Check sheet for the modelled part. Datum: model origin and axes. Units: mm. A direction names the side the tool comes from. Coordinates: 2 decimals unless noted, no trailing zeros. Loops run counter-clockwise (first coordinate to the right, second up) from the corner with the lowest first, then second, coordinate; pieces in that order, holes last.
```python
from build123d import *

# Parameters (mm, degrees)
F0_R     = 6
F1_DEPTH = 16
F2_R     = 2
F3_DEPTH = 12.5
F4_R     = 4
F5_DEPTH = 12


# Not quite as in the source:
# - a fillet or chamfer that OpenCascade refuses, or shapes differently, is made with other operations: its cross-section is extruded or revolved along the edge and cut away or added


with BuildPart() as f1:
    # F0 (on Top) → F1 (new body)
    with BuildSketch(Plane.XY):
        Circle(F0_R)
    extrude(amount=F1_DEPTH)

    # F2 (on Right) → F3 (cut, symmetric)
    with BuildSketch(Plane.YZ):
        with Locations((0, 9.7745376602)):
            Circle(F2_R)
    extrude(amount=F3_DEPTH, both=True, mode=Mode.SUBTRACT)

    # F4 (on face) → F5 (cut)
    with BuildSketch(Plane.XY.offset(16)):
        Circle(F4_R)
    extrude(amount=-F5_DEPTH, mode=Mode.SUBTRACT)

    # F6: fillet of radius 3 on 1 edges, made by hand

    # F6_s1 → F6_t2 (revolve, cut)
    with BuildSketch(Plane.XZ):
        with BuildLine():
            ThreePointArc((6, 13.1715728753), (5.4494897428, 14.9036236828), (4, 16))
            Line((4, 16), (6, 16))
            Line((6, 16), (6, 13.1715728753))
        make_face()
    revolve(axis=Axis((0, 0, 16), (0, 0, 1)), mode=Mode.SUBTRACT)


solid = f1.part
```
1) Depth check by flat-ended pin: pin 1 (3 mm diameter, centred on y = 0, z = 9.77, fed in from +X). Enter the tip coordinate at first touch or a pass-through.
Answer sheet:
pin 1: passes through
2) Section check D-D on z = 6.75. Enter the section's corners in (x, y), plus the area to 3 significant figures.
Answer sheet:
outline: circle Ø12 at (0, 0); hole circle Ø8 at (0, 0)
area: 62.8 mm2
3) Section check B-B on x = 0. Enter the section's corners in (y, z).
Answer sheet:
outline: (-6, 0) - (6, 0) - (6, 13.17) arc R3 ccw to (4, 16) - (4, 4) - (-4, 4) - (-4, 16) arc R3 ccw to (-6, 13.17) - close
4) Mould release check, pull along Z, two halves, no side actions. Record for faces 3 (the cylindrical face through (-4.7, 1.9, 10.4)), 4 (the flat face through (0, 0, 0)), 5 (the flat face through (0, 0, 4)): +Z half, -Z half, draft (parallel to the pull), parting line (faces both ways), or undercut.
Answer sheet:
face 3: undercut
face 4: -Z half
face 5: +Z half
5) Scan lines: line 1 (Y direction, x = 0, z = 10.75); line 2 (Z direction, x = 1.5, y = -2.5); line 3 (Y direction, x = -3.25, z = 11.25). Record each from-to range of solid material in increasing order.
Answer sheet:
line 1: y = -6 to -4, 4 to 6
line 2: z = 0 to 4
line 3: y = -5.04 to -2.33, 2.33 to 5.04
6) Set-up check for faces 1 (the cylindrical face through (5.54, -2.3, 6.49)), 2 (the cylindrical face through (-3.2, -2.4, 10.1)): record each of +Z, -Z, +X, -X, +Y, -Y from which the full face is reachable in a straight line by a thin tool's end or side.
Answer sheet:
face 1: +Z, -Z
face 2: +Z
7) Section check C-C on z = 10.75. Enter the section's corners in (x, y), plus the area to 3 significant figures.
Answer sheet:
outline: (-5.74, -1.75) arc R6 ccw to (5.74, -1.75) - (3.6, -1.75) arc R4 cw to (-3.6, -1.75) - close; (-5.74, 1.75) - (-3.6, 1.75) arc R4 cw to (3.6, 1.75) - (5.74, 1.75) arc R6 ccw to start
area: 48.5 mm2
8) Section check A-A on y = 0. Enter the section's corners in (x, z), plus the area to 3 significant figures.
Answer sheet:
outline: (-6, 0) - (6, 0) - (6, 7.77) - (4, 7.77) - (4, 4) - (-4, 4) - (-4, 7.77) - (-6, 7.77) - close; (-6, 11.77) - (-4, 11.77) - (-4, 16) arc R3 ccw to (-6, 13.17) - close; (4, 11.77) - (6, 11.77) - (6, 13.17) arc R3 ccw to (4, 16) - close
area: 76.9 mm2
